Autodesk Inventor part; units mm, degrees
ref_plane "YZ Plane" through (0, 0, 0) normal (1, 0, 0) x (0, 1, 0)
ref_plane "XZ Plane" through (0, 0, 0) normal (0, 1, 0) x (-1, 0, 0)
ref_plane "XY Plane" through (0, 0, 0) normal (0, 0, 1) x (1, 0, 0)
sketch "Sketch1" plane through (0, 0, 0) normal (0, 0, 1) x (1, 0, 0)
  line L0 (0, 0) -> (0, 10.7581)
  line L1 (1.4, 0) -> (2.1, 0)
  line L2 (2.1, 0) -> (2.4, 0.1732)
  line L3 (2.4, 0.1732) -> (2.4, 4.5)
  line L4 (2.4, 4.5) -> (3, 4.8464)
  line L5 (3, 4.8464) -> (3, 18)
  line L6 (3, 18) -> (1.4, 18)
  line L7 (1.4, 18) -> (1.4, 20.1)
  line L8 (1.4, 20.1) -> (3, 20.1)
  line L9 (3, 20.1) -> (3, 24.7536)
  line L10 (3, 24.7536) -> (2.4, 25.1)
  line L11 (2.4, 25.1) -> (1, 25.1)
  line L12 (1, 25.1) -> (1, 0.4)
  line L13 (1, 0.4) -> (1.4, 0)
  dimension "d0" = 2
  dimension "d1" = 0.4
  dimension "d2" = 0.4
  dimension "d3" = 0.4
  dimension "d4" = 25.1
  dimension "d5" = 20.6
  dimension "d6" = 2.1
  dimension "d7" = 30
  dimension "d8" = 4.2
  dimension "d9" = 4.8
  dimension "d10" = 5
  dimension "d12" = 30
  dimension "d13" = 6
revolve "Revolution1" add sketch "Sketch1" angle 360 about axis through (0, 0, 0) along (0, 1, 0)
thread "Thread1"
thread "Thread2"
equation "\"d3\" = d2"
properties part number "E3D_Heat_Break"
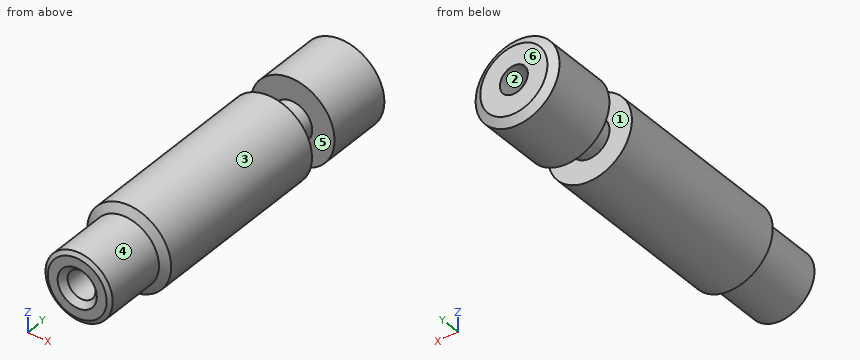
Check sheet for the modelled part. Datum: model origin and axes. Units: mm. Face numbers are marked on the shaded views. A direction names the side the tool comes from. Give positions to 0.01 mm unless a question says otherwise; leave off trailing zeros. Loops run counter-clockwise (first coordinate to the right, second up) from the corner with the lowest first, then second, coordinate; pieces in that order, holes last. Notation, with made-up numbers: M -34.5,-23.75 L 8.5,-23.75 A24 cw 8.5,11.25 Z; hole C 74,-15.75 d1. An arc over 180 degrees is marked long. Use a Markdown table: item, result. Add a question column.
Q1. Sectioned sample at A-A, the plane x = 0. Record the cut outline in (y, z), then the cut area to 3 significant figures.
Q2. Go/stop test with flat-tipped pins: pin 1 (3 mm diameter, centred on x = 0, z = 1.5, fed in from -Y); pin 2 (3 mm diameter, centred on y = 10, z = -2.5, fed in from +X). Record where each tip stops, or that it passes through.
Q3. Sectioned sample at C-C, the plane y = 21.5. Record the cut outline in (x, z).
Q4. Mould release check, pull along X, two halves, no side actions. Record for the marked faces 1, 2 and 3: pulls with the +X half, pulls with the -X half, needs draft (parallel to the pull), parting line crosses it, or undercut.
Q5. Tool access check on the marked faces 4, 5 and 6. Record the directions out of +Z, -Z, +X, -X, +Y, -Y that give a thin tool (end or side, any length) a straight path to the whole face; none if there is none.
Q6. Scan lines: line 1 along Z through (x, y) = (0, 14.75); line 2 along Z through (x, y) = (-0.1, 2.5). Record each from-to range of solid material in increasing order. Write a range as [from, to].
Q7. Sectioned sample at B-B, the plane z = 0. Record the cut outline in (x, y), then the cut area to 3 significant figures.
Verdict:
| question | item | result |
|---|---|---|
| 1 | outline | M 0,-2.1 L 0.17,-2.4 L 4.5,-2.4 L 4.85,-3 L 18,-3 L 18,-1.4 L 20.1,-1.4 L 20.1,-3 L 24.75,-3 L 25.1,-2.4 L 25.1,-1 L 0.4,-1 L 0,-1.4 Z; M 0,1.4 L 0.4,1 L 25.1,1 L 25.1,2.4 L 24.75,3 L 20.1,3 L 20.1,1.4 L 18,1.4 L 18,3 L 4.85,3 L 4.5,2.4 L 0.17,2.4 L 0,2.1 Z |
| 1 | area | 87.7 mm^2 |
| 2 | pin 1 | y = 0 |
| 2 | pin 2 | x = 2.83 |
| 3 | outline | C 0,0 d6; hole C 0,0 d2 |
| 4 | face 1 | needs draft |
| 4 | face 2 | undercut |
| 4 | face 3 | parting line crosses it |
| 5 | face 4 | -Y |
| 5 | face 5 | none |
| 5 | face 6 | +Z, -Z, +X, -X, +Y |
| 6 | line 1 | [-3, -1], [1, 3] |
| 6 | line 2 | [-2.4, -0.99], [0.99, 2.4] |
| 7 | outline | M -3,4.85 L -2.4,4.5 L -2.4,0.17 L -2.1,0 L -1.4,0 L -1,0.4 L -1,25.1 L -2.4,25.1 L -3,24.75 L -3,20.1 L -1.4,20.1 L -1.4,18 L -3,18 Z; M 1,0.4 L 1.4,0 L 2.1,0 L 2.4,0.17 L 2.4,4.5 L 3,4.85 L 3,18 L 1.4,18 L 1.4,20.1 L 3,20.1 L 3,24.75 L 2.4,25.1 L 1,25.1 Z |
| 7 | area | 87.7 mm^2 |
